The listing builds one solid part. Answer for the finished solid, in the listing's coordinates (mm). Face numbers are marked on the shaded views. Round coordinates to 2 decimals unless told otherwise and drop trailing zeros. Loops run counter-clockwise (first coordinate to the right, second up) from the corner with the lowest first, then second, coordinate; pieces in that order, holes last. Notation, with made-up numbers: (61, 74.5) -> (111, 74.5) arc R13 ccw to (111, 80.5) -> close; hole circle Ø8 at (-2, 68). An arc over 180 degrees is marked (long way). Write each question's results on one line, items separated by ' | '. Start each with the question number.
(1) The part is cut by section B-B (z = 19). Determine the outline of the cut face in (x, y).
(2) The part is cut by section A-A (x = 3.25). Determine the outline of the cut face in (y, z).
(3) Straight lines are drawn through the part: probe 1 along Y at (x, z) = (3.45, 21.5); probe 2 along Y at (x, z) = (1.4, 19.5); probe 3 along Y at (x, z) = (2.4, 24.25). For each, find the intervals that lie inside material, in ascending order.
(4) The part is cut by section C-C (z = 24.5). Determine the outline of the cut face in (x, y).
(5) The part is cut by section D-D (z = 16.5). Determine the outline of the cut face in (x, y).
(6) Determine the mould class of the marked faces 1 and 2 for opening direction Y: released by +Y, released by -Y, zero draft, split by the parting line, or undercut.
(7) A flat-ended cylindrical pin translates along its axis: pin 1 (3.5 mm diameter, centred on y = -12.01, z = 20.33, fed in from -X). Find the tip coordinate at first contact, or state that the pin passes through.
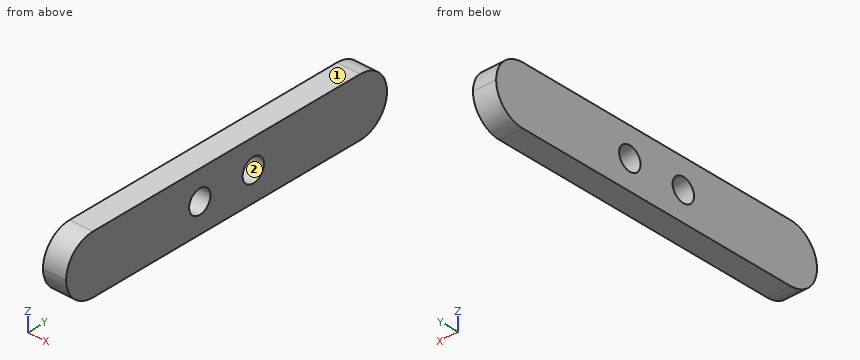
```python
from build123d import *

# Parameters (mm, degrees)
F1_DEPTH = 4
F2_R     = 2
F3_DEPTH = 25


with BuildPart() as f1:
    # F0 (on Right) → F1 (new body)
    with BuildSketch(Plane.YZ):
        with BuildLine():
            Line((17.990056, 25.330209), (-32.009944, 25.330209))
            ThreePointArc((-32.009944, 25.330209), (-35.545478, 23.865743), (-37.009944, 20.330209))
            ThreePointArc((-37.009944, 20.330209), (-35.545478, 16.794676), (-32.009944, 15.330209))
            Line((-32.009944, 15.330209), (17.990056, 15.330209))
            ThreePointArc((17.990056, 15.330209), (21.52559, 16.794676), (22.990056, 20.330209))
            ThreePointArc((22.990056, 20.330209), (21.52559, 23.865743), (17.990056, 25.330209))
        make_face()
    extrude(amount=F1_DEPTH)

    # F2 (on face) → F3 (cut)
    with BuildSketch(Plane.YZ.offset(4)):
        with Locations((-12.009944, 20.330209)):
            Circle(F2_R)
        with Locations((-2.009944, 20.330209)):
            Circle(F2_R)
    extrude(amount=-F3_DEPTH, mode=Mode.SUBTRACT)


solid = f1.part
```
Checked values:
1) outline: (0, -36.83) -> (4, -36.83) -> (4, -13.5) -> (0, -13.5) -> close; (0, -10.52) -> (4, -10.52) -> (4, -3.5) -> (0, -3.5) -> close; (0, -0.52) -> (4, -0.52) -> (4, 22.81) -> (0, 22.81) -> close
2) outline: (-37.01, 20.33) arc R5 ccw to (-32.01, 15.33) -> (17.99, 15.33) arc R5 ccw to (22.99, 20.33) arc R5 ccw to (17.99, 25.33) -> (-32.01, 25.33) arc R5 ccw to start; hole circle Ø4 at (-12.01, 20.33); hole circle Ø4 at (-2.01, 20.33)
3) probe 1: y = -36.87 to -13.63, -10.39 to -3.63, -0.39 to 22.85 | probe 2: y = -36.94 to -13.83, -10.19 to -3.83, -0.19 to 22.92 | probe 3: y = -35.11 to 21.09
4) outline: (0, -34.77) -> (4, -34.77) -> (4, 20.75) -> (0, 20.75) -> close
5) outline: (0, -35.22) -> (4, -35.22) -> (4, 21.2) -> (0, 21.2) -> close
6) face 1: zero draft | face 2: undercut
7) pin 1: passes through
